Autodesk Inventor part; units mm, degrees
ref_plane "YZ Plane" through (0, 0, 0) normal (1, 0, 0) x (0, 1, 0)
ref_plane "XZ Plane" through (0, 0, 0) normal (0, 1, 0) x (-1, 0, 0)
ref_plane "XY Plane" through (0, 0, 0) normal (0, 0, 1) x (1, 0, 0)
sketch "Sketch1" plane through (0, 0, 0) normal (0, 1, 0) x (-1, 0, 0)
  line L0 (0, 0) -> (105.41, 0)
  line L1 (105.41, 0) -> (105.41, 863.6)
  line L2 (105.41, 863.6) -> (0, 863.6)
  line L3 (0, 863.6) -> (0, 0)
  dimension "d0" = 105.41
  dimension "d1" = 863.6
extrude "Extrusion1" add sketch "Sketch1" along normal blind 12.7
sketch "Sketch2" plane through (0, 12.7, 0) normal (0, 1, 0) x (1, 0, 0)
  line L0 (0, 0) -> (-105.41, 0)
  line L1 (0, 0) -> (-12.7, 0)
  line L2 (-12.7, 0) -> (-12.7, 12.7)
  line L3 (-12.7, 12.7) -> (0, 12.7)
  line L4 (0, 12.7) -> (0, 0)
  line L5 (-105.41, 0) -> (-105.41, -863.6)
  line L6 (0, 12.7) -> (-105.41, 12.7)
  line L7 (-105.41, 12.7) -> (-105.41, 0)
  line L8 (-105.41, 0) -> (0, 0)
  line L9 (0, 0) -> (0, 12.7)
  line L10 (0, -863.6) -> (0, 0)
  line L11 (0, -863.6) -> (-105.41, -863.6)
  line L12 (-105.41, -863.6) -> (-105.41, -876.3)
  line L13 (-105.41, -876.3) -> (0, -876.3)
  line L14 (0, -876.3) -> (0, -863.6)
  line L15 (-105.41, -863.6) -> (-92.71, -863.6)
  line L16 (-92.71, -863.6) -> (-92.71, 12.7)
  line L17 (-92.71, 12.7) -> (-105.41, 12.7)
  line L18 (-105.41, 12.7) -> (-105.41, -863.6)
  line L19 (0, 12.7) -> (-12.7, 12.7)
  line L20 (-12.7, 12.7) -> (-12.7, -876.3)
  line L21 (-12.7, -876.3) -> (0, -876.3)
  line L22 (0, -876.3) -> (0, 12.7)
  point P0 (-12.7, -863.6)
  point P1 (-92.71, 0)
  dimension "d4" = 12.7
  dimension "d5" = 12.7
  dimension "d6" = 12.7
  dimension "d7" = 12.7
  dimension "d8" = 12.7
extrude "Extrusion2" add sketch "Sketch2" along normal blind 95.25 and the other way blind 12.7 contours L10 L11 L20 L0 | L0 L2 L3 L4 | L0 L16 L6 L2 | L14 L13 L20 L11 | L16 L11 L5 L0 | L0 L7 L6 L16 | L20 L13 L12 L11
sketch "Sketch3" plane through (-105.41, 107.95, 876.3) normal (0, 0, 1) x (1, 0, 0)
  line L0 (12.7, -95.25) -> (92.71, -95.25)
  line L1 (12.7, -95.25) -> (12.7, 0)
  line L2 (92.71, -95.25) -> (92.71, 0)
  line L3 (92.71, -95.25) -> (77.47, -95.25)
  line L4 (77.47, -95.25) -> (77.47, -12.7)
  line L5 (77.47, -12.7) -> (92.71, -12.7)
  line L6 (92.71, -12.7) -> (92.71, -95.25)
  line L7 (12.7, -95.25) -> (27.94, -95.25)
  line L8 (27.94, -95.25) -> (27.94, -12.7)
  line L9 (27.94, -12.7) -> (12.7, -12.7)
  line L10 (12.7, -12.7) -> (12.7, -95.25)
  line L11 (27.94, -95.25) -> (34.29, -95.25)
  line L12 (34.29, -95.25) -> (34.29, -12.7)
  line L13 (34.29, -12.7) -> (27.94, -12.7)
  line L14 (27.94, -12.7) -> (27.94, -95.25)
  line L15 (77.47, -95.25) -> (71.12, -95.25)
  line L16 (71.12, -95.25) -> (71.12, -12.7)
  line L17 (71.12, -12.7) -> (77.47, -12.7)
  line L18 (77.47, -12.7) -> (77.47, -95.25)
  line L19 (34.29, -95.25) -> (49.53, -95.25)
  line L20 (49.53, -95.25) -> (49.53, -12.7)
  line L21 (49.53, -12.7) -> (34.29, -12.7)
  line L22 (34.29, -12.7) -> (34.29, -95.25)
  line L23 (71.12, -95.25) -> (55.88, -95.25)
  line L24 (55.88, -95.25) -> (55.88, -12.7)
  line L25 (55.88, -12.7) -> (71.12, -12.7)
  line L26 (71.12, -12.7) -> (71.12, -95.25)
  point P0 (105.41, -107.95)
  dimension "d13" = 15.24
  dimension "d14" = 82.55
  dimension "d15" = 15.24
  dimension "d16" = 6.35
  dimension "d17" = 6.35
  dimension "d18" = 15.24
  dimension "d19" = 15.24
extrude "Extrusion3" cut sketch "Sketch3" against normal blind 95.25 contours L1 L9 L8 L0 | L24 L25 L16 L0 | L12 L21 L20 L0 | L4 L5 L2 L0
sketch "Sketch5" plane through (-105.41, 107.95, 876.3) normal (0, 0, 1) x (1, 0, 0)
  line L0 (71.12, -95.25) -> (55.88, -95.25)
  line L1 (55.88, -95.25) -> (55.88, -12.7)
  line L2 (55.88, -12.7) -> (71.12, -12.7)
  line L3 (71.12, -12.7) -> (71.12, -95.25)
  line L4 (49.53, -95.25) -> (34.29, -95.25)
  line L5 (34.29, -95.25) -> (34.29, -12.7)
  line L6 (34.29, -12.7) -> (49.53, -12.7)
  line L7 (49.53, -12.7) -> (49.53, -95.25)
  line L8 (92.71, -95.25) -> (77.47, -95.25)
  line L9 (77.47, -95.25) -> (77.47, -12.7)
  line L10 (77.47, -12.7) -> (92.71, -12.7)
  line L11 (92.71, -12.7) -> (92.71, -95.25)
  line L12 (27.94, -95.25) -> (12.7, -95.25)
  line L13 (12.7, -95.25) -> (12.7, -12.7)
  line L14 (12.7, -12.7) -> (27.94, -12.7)
  line L15 (27.94, -12.7) -> (27.94, -95.25)
  line L16 (105.41, -107.95) -> (105.41, 0)
  line L17 (0, 0) -> (105.41, 0)
  line L18 (0, -107.95) -> (0, 0)
  line L19 (105.41, -107.95) -> (0, -107.95)
  line L20 (92.71, 0) -> (12.7, 0)
  circle A0 centre (52.705, 26.3525) radius 26.3525
  dimension "d40" = 52.705
extrude "Extrusion4" add sketch "Sketch5" against normal blind 1270 contours A0
sketch "Sketch6" plane through (0, 0, -12.7) normal (1, 0, 0) x (0, 0, -1)
  line L0 (0, 0) -> (-889, 0)
  line L1 (-444.5, 0) -> (-444.5, 160.655)
  line L2 (-889, 160.655) -> (381, 160.655)
  line L3 (-444.5, 160.655) -> (-444.5, 167.005)
  line L4 (-444.5, 0) -> (-444.5, -6.35)
  line L5 (-444.5, 167.005) -> (-428.625, 167.005)
  line L6 (-428.625, 167.005) -> (-460.375, 167.005)
  line L7 (-428.625, 167.005) -> (-460.375, 167.005)
  line L8 (-460.375, 167.005) -> (-460.375, -6.35)
  line L9 (-460.375, -6.35) -> (-428.625, -6.35)
  line L10 (-428.625, -6.35) -> (-428.625, 167.005)
  line L11 (-889, 0) -> (-793.75, 0)
  line L12 (0, 107.95) -> (0, 0)
  line L13 (0, 0) -> (-95.25, 0)
  line L14 (-95.25, 0) -> (-95.25, -6.35)
  line L15 (-793.75, 0) -> (-793.75, -6.35)
  line L16 (-793.75, -6.35) -> (-762, -6.35)
  line L17 (-762, -6.35) -> (-762, 167.005)
  line L18 (-762, 167.005) -> (-793.75, 167.005)
  line L19 (-793.75, 167.005) -> (-793.75, -6.35)
  line L20 (-95.25, -6.35) -> (-127, -6.35)
  line L21 (-127, -6.35) -> (-127, 167.005)
  line L22 (-127, 167.005) -> (-95.25, 167.005)
  line L23 (-95.25, 167.005) -> (-95.25, -6.35)
  line L24 (-111.125, 167.005) -> (-111.125, -6.35)
  line L25 (-777.875, -6.35) -> (-777.875, 167.005)
  line L26 (-777.875, 79.2503) -> (-762, 79.2503)
  line L27 (-111.125, 68.9503) -> (-95.25, 68.9503)
  line L28 (-451.8389, 167.005) -> (-451.8389, 163.0426)
  circle A0 centre (-444.5, 148.7424) radius 10.8761
  circle A1 centre (-444.5, 11.9126) radius 11.9126
  line L29 (-456.4123, 12.0028) -> (-455.3758, 148.8248)
  line L30 (-433.6242, 148.8248) -> (-432.5877, 12.0028)
  line L31 (-127, 12.7) -> (-139.7, 12.7)
  line L32 (-139.7, 12.7) -> (-165.1, 12.7)
  line L33 (-460.375, 21.426) -> (-473.075, 21.426)
  line L34 (0, 107.95) -> (-889, 107.95)
  line L35 (-524.7767, 107.95) -> (-524.7767, 0)
  line L36 (-524.7767, 53.975) -> (-485.775, 53.975)
  circle A2 centre (-485.775, 53.975) radius 12.7
  line L37 (-498.475, 0) -> (-498.475, -3.175)
  line L38 (-498.475, -3.175) -> (-473.075, -3.175)
  line L39 (-473.075, -3.175) -> (-473.075, 53.975)
  line L40 (-498.475, 53.975) -> (-498.475, 0)
  line L41 (-694.0635, 0) -> (-694.0635, 19.05)
  line L42 (-762, 19.05) -> (-571.5, 19.05)
  line L43 (-687.1312, 19.05) -> (-687.1312, 44.45)
  line L44 (-762, 44.45) -> (-565.15, 44.45)
  line L45 (-571.5, 19.05) -> (-565.15, 44.45)
  point P0 (-12.7, 0)
  dimension "d25" = 6.35
  dimension "d26" = 6.35
  dimension "d27" = 15.875
  dimension "d28" = 31.75
  dimension "d29" = 95.25
  dimension "d30" = 95.25
  dimension "d31" = 6.35
  dimension "d32" = 6.35
  dimension "d33" = 31.75
  dimension "d34" = 31.75
  dimension "d35" = 3.9624
  dimension "d39" = 23.8252
  dimension "d41" = 12.7
  dimension "d42" = 25.4
  dimension "d43" = 12.7
  dimension "d45" = 19.05
  dimension "d46" = 190.5
  dimension "d47" = 25.4
  dimension "d48" = 196.85
sketch "Sketch7" plane through (-105.41, 0, 876.3) normal (0, 0, 1) x (1, 0, 0)
  point P0 (105.41, 0)
extrude "Extrusion5" cut sketch "Sketch6" against normal blind 15.24 contours L42 L17 L44 L43 | L43 L44 L45 L42
sketch "Sketch8" plane through (0, 107.95, 0) normal (0, 1, 0) x (1, 0, 0)
  line L0 (0, -876.3) -> (0, 12.7)
  line L1 (-105.41, 12.7) -> (-105.41, -876.3)
  line L2 (0, 12.7) -> (-105.41, 12.7)
  line L3 (-105.41, 12.7) -> (-105.41, -876.3)
  line L4 (-105.41, -876.3) -> (0, -876.3)
  line L5 (0, -876.3) -> (0, 12.7)
  point P0 (0, 0)
extrude "Extrusion6" add sketch "Sketch8" against normal blind 12.7
sketch "Sketch9" plane through (-52.705, 134.3025, 876.3) normal (0, 0, 1) x (1, 0, 0)
  line L0 (-52.705, -26.3525) -> (0, -26.3525)
  line L1 (-39.5109, -26.3525) -> (301.585, -26.3525)
  line L2 (301.585, -26.3525) -> (301.585, 239.994)
  line L3 (301.585, 239.994) -> (-39.5109, 239.994)
  line L4 (-39.5109, 239.994) -> (-39.5109, -26.3525)
  point P0 (52.705, -134.3025)
extrude "Extrusion7" cut sketch "Sketch9" against normal through all
sketch "Sketch10" plane through (-105.41, 0, 876.3) normal (0, 0, 1) x (1, 0, 0)
  point P0 (105.41, 0)
properties part number "box"
CAD build for the part. Positions are in the model's coordinates, mm. A direction names the side the tool comes from. Coordinates: 2 decimals unless noted, no trailing zeros. Loops run counter-clockwise (first coordinate to the right, second up) from the corner with the lowest first, then second, coordinate; pieces in that order, holes last. Notation, with made-up numbers: (-10, 55.5) - (46, 55.5) arc R28 ccw to (46, 87.5) - close; hole circle Ø8 at (73.5, 61). An arc over 180 degrees is marked (long way). Use one line per item in the form item = value. Start each with the question number.
1) Band-saw the part on A-A (y = 63.5). Give the cut face in (x, z).
2) Tool access for faces 1 (the face through (-53, 107.95, 426)), 2 (the face through (-92.71, 53, 444)): list every direction of +Z, -Z, +X, -X, +Y, -Y with a clear straight run to the whole face (end or side of a thin tool).
3) Band-saw the part on C-C (y = 27). Give the cut face in (x, z).
4) Band-saw the part on D-D (x = -63.5). Give the cut face in (y, z).
5) Band-saw the part on B-B (z = 153.5). Give the cut face in (x, y).
6) Drill centre lines: L1, parallel to Y at x = -78.5, z = 264; L2, parallel to X at y = 90, z = 823.5; L3, parallel to Z at x = -34, y = 23. Where is each one in solid material? Low to high. Write a range as from..to.
7) Flat gauge pin, fed straight in: pin 1 (3 mm diameter, centred on x = -65, y = 65.5, fed in from +Z). Where does the tip first touch, or does it go through?
Check values:
q1.outline = (-105.41, -12.7) - (0, -12.7) - (0, 876.3) - (-12.7, 876.3) - (-12.7, 0) - (-92.71, 0) - (-92.71, 876.3) - (-105.41, 876.3) - close; (-77.47, 863.6) - (-71.12, 863.6) - (-71.12, 876.3) - (-77.47, 876.3) - close; (-55.88, 863.6) - (-49.53, 863.6) - (-49.53, 876.3) - (-55.88, 876.3) - close; (-34.29, 863.6) - (-27.94, 863.6) - (-27.94, 876.3) - (-34.29, 876.3) - close
q2.face_1 = +Z, -Z, +X, -X, +Y
q2.face_2 = +Z
q3.outline = (-105.41, -12.7) - (0, -12.7) - (0, 556.81) - (-12.7, 556.81) - (-12.7, 0) - (-92.71, 0) - (-92.71, 876.3) - (-105.41, 876.3) - close; (-77.47, 863.6) - (-71.12, 863.6) - (-71.12, 876.3) - (-77.47, 876.3) - close; (-55.88, 863.6) - (-49.53, 863.6) - (-49.53, 876.3) - (-55.88, 876.3) - close; (-34.29, 863.6) - (-27.94, 863.6) - (-27.94, 876.3) - (-34.29, 876.3) - close; (-12.7, 749.3) - (0, 749.3) - (0, 876.3) - (-12.7, 876.3) - close
q4.outline = (0, -12.7) - (107.95, -12.7) - (107.95, 876.3) - (95.25, 876.3) - (95.25, 0) - (12.7, 0) - (12.7, 876.3) - (0, 876.3) - close
q5.outline = (-105.41, 0) - (0, 0) - (0, 107.95) - (-105.41, 107.95) - close; hole (-92.71, 12.7) - (-12.7, 12.7) - (-12.7, 95.25) - (-92.71, 95.25) - close
q6.L1 = 0..12.7, 95.25..107.95
q6.L2 = -105.41..-92.71, -12.7..0
q6.L3 = -12.7..0, 863.6..876.3
q7.pin_1 = 0
